```python
from build123d import *

# Parameters (mm, degrees)
F0_R        = 5
F0_R_2      = 4
F3_C1_SIZE2 = 0.6516126864
F3_C1_SIZE  = 0.5
F3_C2_SIZE2 = 0.5
F3_C2_SIZE  = 0.6516126864


with BuildPart() as f2:
    # F2: sweep along a path in F1
    with BuildLine(Plane.XZ) as f2_path:
        Line((0, 0), (0, 21))
        ThreePointArc((0, 21), (-5.2720779386, 33.7279220614), (-18, 39))
        Line((-18, 39), (-47, 39))
        ThreePointArc((-47, 39), (-59.7279220614, 44.2720779386), (-65, 57))
        Line((-65, 57), (-65, 70))
    # F0 (on Top) → F2 (sweep)
    with BuildSketch(Plane.XY):
        Circle(F0_R)
        Circle(F0_R_2, mode=Mode.SUBTRACT)
    sweep(path=f2_path.line)

    # F3: chamfer of 0.5 x 0.6516126864 on 2 edges, made by hand

    # F3_c1
    f3_c1_edges = [f2.edges().sort_by_distance(p)[0] for p in [
        (-5, 0, 0),
    ]]
    f3_c1_side = f2.faces().sort_by_distance((-5, 0, 0.01))[0]
    chamfer(f3_c1_edges, length=F3_C1_SIZE, length2=F3_C1_SIZE2, reference=f3_c1_side)

    # F3_c2
    f3_c2_edges = [f2.edges().sort_by_distance(p)[0] for p in [
        (-70, 0, 70),
    ]]
    f3_c2_side = f2.faces().sort_by_distance((-70, 0, 69.99))[0]
    chamfer(f3_c2_edges, length=F3_C2_SIZE, length2=F3_C2_SIZE2, reference=f3_c2_side)


solid = f2.part
```
Work out the finished part from the listing and answer in its coordinate system (mm). A direction names the side the tool comes from. Give positions to 0.01 mm unless a question says otherwise; leave off trailing zeros. Write each loop counter-clockwise with the first axis right and the second up, starting at its lowest first coordinate (ties: lowest second). Pieces come first, ordered by that corner, then holes.
(1) The part is cut by section B-B on x = -31. Write down the section's boundary in (y, z), plus the area to 3 significant figures.
Final values:
outline: circle Ø10 at (0, 39); hole circle Ø8 at (0, 39)
area: 28.3 mm2
(2) Flat-ended cylindrical pins translate along their axes: pin 1 Ø1 at (x, y) = (-10, -2.5) entering from -Z; pin 2 Ø2 at (x, z) = (-61, 51) entering from +Y; pin 3 Ø5 at (y, z) = (0, 39) entering from +X. Find the tip coordinate at first contact, or state that the pin passes through.
Final values:
pin 1: stops at z = 31.58
pin 2: stops at y = 4.68
pin 3: stops at x = -1.01
(3) Which of the six approach directions +Z, -Z, +X, -X, +Y, -Y give full straight-line access (tool end or side, diameter ignored) to faces 5 (the cylindrical face through (-1.08, -4.88, 10.89)), 6 (the cylindrical face through (-70, 0, 63))?
Final values:
face 5: -Z
face 6: +Z
(4) The part is cut by section A-A on y = 0. Write down the section's boundary in (x, z), plus the area to 3 significant figures.
Final values:
outline: (-70, 57) arc R23 ccw to (-47, 34) - (-18, 34) arc R13 cw to (-5, 21) - (-5, 0.5) - (-4.35, 0) - (-4, 0) - (-4, 21) arc R14 ccw to (-18, 35) - (-47, 35) arc R22 cw to (-69, 57) - (-69, 70) - (-69.5, 70) - (-70, 69.35) - close; (-61, 57) arc R14 ccw to (-47, 43) - (-18, 43) arc R22 cw to (4, 21) - (4, 0) - (4.35, 0) - (5, 0.5) - (5, 21) arc R23 ccw to (-18, 44) - (-47, 44) arc R13 cw to (-60, 57) - (-60, 69.35) - (-60.5, 70) - (-61, 70) - close
area: 238 mm2
(5) Straight lines are drawn through the part: line 1 (Y direction, x = -32.5, z = 39); line 2 (Z direction, x = -29.75, y = 0); line 3 (Z direction, x = -50, y = -0.5). For each, find the intervals that lie inside material, in ascending order.
Final values:
line 1: y = -5 to -4, 4 to 5
line 2: z = 34 to 35, 43 to 44
line 3: z = 34.22 to 35.24, 43.29 to 44.33
(6) The mould has two halves that part along Z. Classify faces 1 (the cylindrical face through (-32.7, -2.4, 35.8)), 2 (the flat face through (-68, -3, 70)), 3 (the cylindrical face through (-33, 0, 34)), 4 (the cylindrical face through (-0.867, -3.905, 10.647)): pulls with the +Z half, pulls with the -Z half, needs draft (parallel to the pull), parting line crosses it, or undercut.
Final values:
face 1: undercut
face 2: pulls with the +Z half
face 3: parting line crosses it
face 4: needs draft
